Job drawing, mm, ordinate dimensions from the low corner. One solid piece. Round coordinates to 2 decimals unless told otherwise and drop trailing zeros. Loops run counter-clockwise (first coordinate to the right, second up) from the corner with the lowest first, then second, coordinate; pieces in that order, holes last. Notation, with made-up numbers: (74, -32.75) - (120, -32.75) arc R23 ccw to (120, -15.75) - close; hole circle Ø4 at (39, 36). An arc over 180 degrees is marked (long way). Answer as CSV lines item,"result". Start each with the question number.
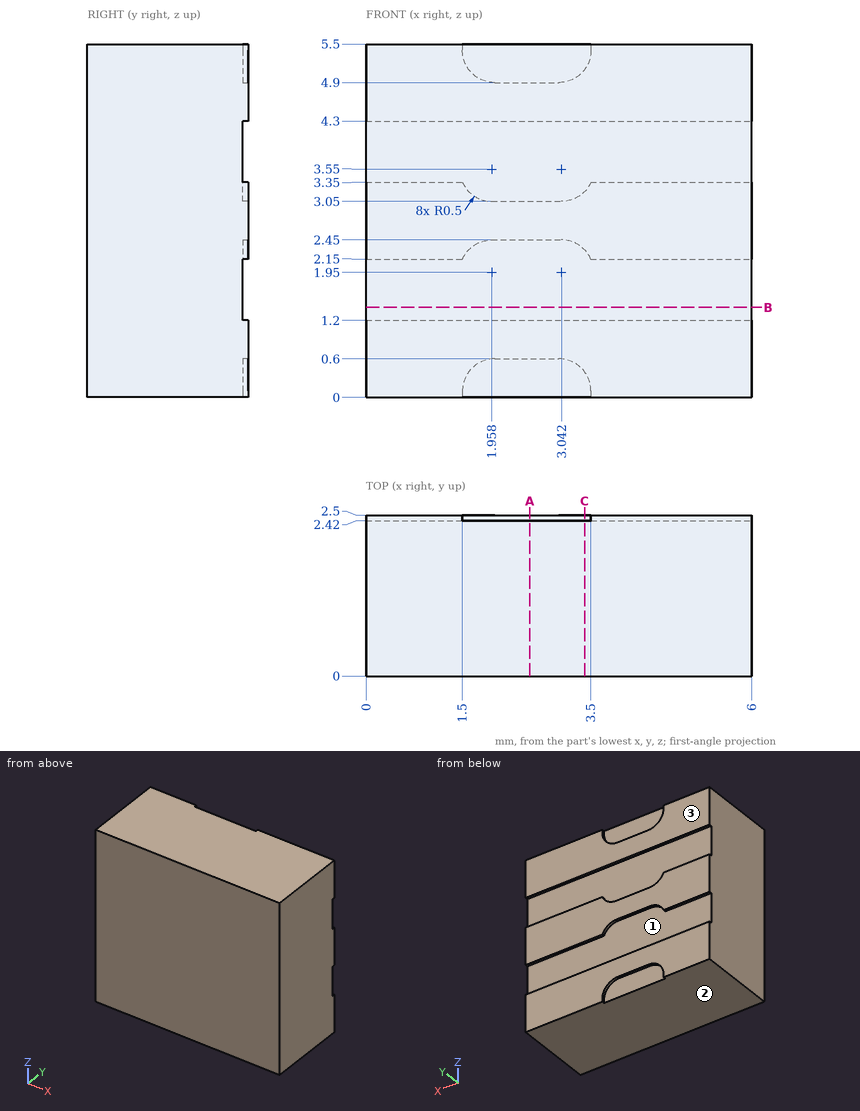
Q1. Wall check: probe 1 along Y at (x, z) = (3.3, 3.35). Give the ranges that are in metal, low to high. Write a range as [from, to].
Q2. Two-plate mould, pull along Z, no slides. Class the marked faces 1, 2 and 3: released by +Z, released by -Z, zero draft, split by the parting line, or undercut.
Q3. Band-saw the part on A-A, the plane x = 2.55. List the corners of the cut face in (y, z).
Q4. Band-saw the part on C-C, the plane x = 3.4. List the corners of the cut face in (y, z), then the cut area to 3 significant figures.
Q5. Band-saw the part on B-B, the plane z = 1.4. List the corners of the cut face in (x, y).
Reported:
1,probe 1,"y = [0, 2.42]"
2,face 1,"undercut"
2,face 2,"released by -Z"
2,face 3,"zero draft"
3,outline,"(0, 0) - (2.42, 0) - (2.42, 0.6) - (2.5, 0.6) - (2.5, 1.2) - (2.42, 1.2) - (2.42, 2.45) - (2.5, 2.45) - (2.5, 3.05) - (2.42, 3.05) - (2.42, 4.3) - (2.5, 4.3) - (2.5, 4.9) - (2.42, 4.9) - (2.42, 5.5) - (0, 5.5) - close"
4,outline,"(0, 0) - (2.42, 0) - (2.42, 0.4) - (2.5, 0.4) - (2.5, 1.2) - (2.42, 1.2) - (2.42, 2.3) - (2.5, 2.3) - (2.5, 3.2) - (2.42, 3.2) - (2.42, 4.3) - (2.5, 4.3) - (2.5, 5.1) - (2.42, 5.1) - (2.42, 5.5) - (0, 5.5) - close"
4,area,"13.5 mm2"
5,outline,"(0, 0) - (6, 0) - (6, 2.42) - (0, 2.42) - close"
